Here's how the part is built. I have some questions about the finished solid (model axes, mm). Face numbers are marked on the shaded views. A direction names the side the tool comes from. Round coordinates to 2 decimals unless told otherwise and drop trailing zeros. Loops run counter-clockwise (first coordinate to the right, second up) from the corner with the lowest first, then second, coordinate; pieces in that order, holes last. Notation, with made-up numbers: (-17, 28) -> (3, 28) arc R37 cw to (3, 66) -> close; hole circle Ø8 at (66, 2). An arc over 180 degrees is marked (long way). Use CSV: the item, a comma, the result in double quotes. Start each with the question number.
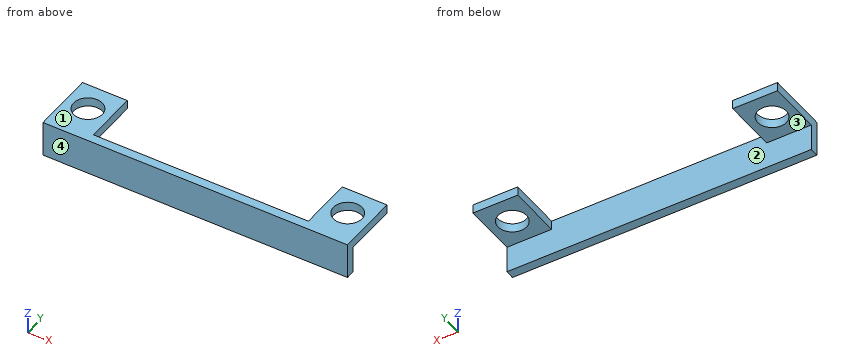
from build123d import *

# Parameters (mm, degrees)
SKETCH1_W           = 34
SKETCH1_H           = 4
BOSS_EXTRUDE1_DEPTH = 1
SKETCH2_W           = 5
SKETCH2_H           = 1
BOSS_EXTRUDE2_DEPTH = 6
SKETCH3_R           = 1.6
CUT_EXTRUDE1_DEPTH  = 6


with BuildPart() as part:
    # Sketch1 → Boss-Extrude1 (new body)
    with BuildSketch(Plane(origin=(0, 0, 0), x_dir=(1, 0, 0), z_dir=(0, 1, 0))):
        Rectangle(SKETCH1_W, SKETCH1_H)
    extrude(amount=BOSS_EXTRUDE1_DEPTH)

    # Sketch2 → Boss-Extrude2 (add)
    with BuildSketch(Plane(origin=(0, 1, 0), x_dir=(1, 0, 0), z_dir=(0, 1, 0))):
        with Locations((-14.5, -1.5)):
            Rectangle(SKETCH2_W, SKETCH2_H)
        with Locations((14.5, -1.5)):
            Rectangle(SKETCH2_W, SKETCH2_H)
    extrude(amount=BOSS_EXTRUDE2_DEPTH)

    # Sketch3 → Cut-Extrude1 (cut)
    with BuildSketch(Plane.XY.offset(2)):
        with Locations((-14.5, 4)):
            Circle(SKETCH3_R)
        with Locations((14.5, 4)):
            Circle(SKETCH3_R)
    extrude(amount=-CUT_EXTRUDE1_DEPTH, mode=Mode.SUBTRACT)


solid = part.part
Q1. I want a section at A-A, the plane x = -14.5. List the corners of the cut face in (y, z) for me.
Q2. I need wall thicknesses on line 1 along Y through (x, z) = (14.5, 1.45); line 2 along Y through (x, z) = (-3.5, -1.05); line 3 along X through (y, z) = (2, 1.1). Which ranges of each line are inside material? Lowest first, please.
Q3. I want a section at D-D, the plane x = 13.5. List the corners of the cut face in (y, z) for me.
Q4. Will these pins go through, and if not, where does the flat tip stop? pin 1 Ø3 at (x, y) = (5.5, 3) entering from +Z; pin 2 Ø4 at (x, y) = (9, 1.5) entering from -Z; pin 3 Ø2 at (x, z) = (-2, 0) entering from +Y; pin 4 Ø3.5 at (x, y) = (14.5, 4) entering from -Z.
Q5. For the marked faces 3 and 4, which set-ups out of +Z, -Z, +X, -X, +Y, -Y let a thin tool reach every point of the face, with its end or its side?
Q6. I want a section at C-C, the plane z = -1.7. List the corners of the cut face in (x, y) for me, then the cut area to 3 significant figures.
Q7. If we mould it in two halves opening along X, with no side actions, what happens to the marked faces 1 and 2? For each: pulls with the +X half, pulls with the -X half, needs draft (parallel to the pull), parting line crosses it, or undercut.
Q8. I want a section at B-B, the plane y = 4. List the corners of the cut face in (x, z) for me.
Values found:
1,outline,"(0, -2) -> (1, -2) -> (1, 1) -> (2.4, 1) -> (2.4, 2) -> (0, 2) -> close; (5.6, 1) -> (7, 1) -> (7, 2) -> (5.6, 2) -> close"
2,line 1,"0 to 2.4, 5.6 to 7"
2,line 2,"0 to 1"
2,line 3,"-17 to -12, 12 to 17"
3,outline,"(0, -2) -> (1, -2) -> (1, 1) -> (2.75, 1) -> (2.75, 2) -> (0, 2) -> close; (5.25, 1) -> (7, 1) -> (7, 2) -> (5.25, 2) -> close"
4,pin 1,"through"
4,pin 2,"z = -2"
4,pin 3,"y = 1"
4,pin 4,"z = 1"
5,face 3,"-Z, +X, -X, +Y"
5,face 4,"+Z, -Z, +X, -X, -Y"
6,outline,"(-17, 0) -> (17, 0) -> (17, 1) -> (-17, 1) -> close"
6,area,"34.0 mm2"
7,face 1,"needs draft"
7,face 2,"undercut"
8,outline,"(-17, 1) -> (-16.1, 1) -> (-16.1, 2) -> (-17, 2) -> close; (-12.9, 1) -> (-12, 1) -> (-12, 2) -> (-12.9, 2) -> close; (12, 1) -> (12.9, 1) -> (12.9, 2) -> (12, 2) -> close; (16.1, 1) -> (17, 1) -> (17, 2) -> (16.1, 2) -> close"
